Geometry: final body of the model. Coordinates: model frame, mm. Give positions to 0.01 mm unless a question says otherwise; leave off trailing zeros. Order: outer loops, then holes, each group sorted by start corner. A loop starts at its lowest first (then second) coordinate and runs counter-clockwise, first axis right, second up. Notation, with made-up numbers: (26.5, 1) -> (66.5, 1) arc R36 cw to (66.5, 40) -> close; hole circle Ø1 at (-0.5, -10). An arc over 180 degrees is marked (long way). One line per question, with ' | ' between items.
from build123d import *

# Parameters (mm, degrees)
SKETCH_1_R      = 1.65
EXTRUDE_1_DEPTH = 5
FILLET_1_R      = 2


with BuildPart() as part:
    # ｽｹｯﾁ1 → ﾎﾞｽ - 押し出し1 (new body)
    with BuildSketch(Plane.XY):
        Polygon((0, 0), (40, 0), (40, 15), (15, 60), (0, 60), align=None)
        with Locations((35, 7.5)):
            Circle(SKETCH_1_R, mode=Mode.SUBTRACT)
        with Locations((7.5, 7.5)):
            Circle(SKETCH_1_R, mode=Mode.SUBTRACT)
        with Locations((7.5, 22.5)):
            Circle(SKETCH_1_R, mode=Mode.SUBTRACT)
        with Locations((7.5, 52.5)):
            Circle(SKETCH_1_R, mode=Mode.SUBTRACT)
    extrude(amount=EXTRUDE_1_DEPTH)

    # ﾌｨﾚｯﾄ1
    fillet_1_edges = [part.edges().sort_by_distance(p)[0] for p in [
        (0, 60, 2.5),
        (15, 60, 2.5),
        (40, 15, 2.5),
        (40, 0, 2.5),
        (0, 0, 2.5),
    ]]
    fillet(fillet_1_edges, radius=FILLET_1_R)


solid = part.part
1) Section B-B on z = 2.55. Return loops of the section in (x, y), plus the area to 3 significant figures.
Check result:
outline: (0, 2) arc R2 ccw to (2, 0) -> (38, 0) arc R2 ccw to (40, 2) -> (40, 14.48) arc R2 ccw to (39.75, 15.45) -> (15.57, 58.97) arc R2 ccw to (13.82, 60) -> (2, 60) arc R2 ccw to (0, 58) -> close; hole circle Ø3.3 at (7.5, 7.5); hole circle Ø3.3 at (7.5, 22.5); hole circle Ø3.3 at (7.5, 52.5); hole circle Ø3.3 at (35, 7.5) | area: 1,800 mm^2
2) Section D-D on y = 22.5. Return loops of the section in (x, z), plus the area to 3 significant figures.
Check result:
outline: (0, 0) -> (5.85, 0) -> (5.85, 5) -> (0, 5) -> close; (9.15, 0) -> (35.83, 0) -> (35.83, 5) -> (9.15, 5) -> close | area: 163 mm^2
3) Section A-A on x = 7.5. Return loops of the section in (y, z).
Check result:
outline: (0, 0) -> (5.85, 0) -> (5.85, 5) -> (0, 5) -> close; (9.15, 0) -> (20.85, 0) -> (20.85, 5) -> (9.15, 5) -> close; (24.15, 0) -> (50.85, 0) -> (50.85, 5) -> (24.15, 5) -> close; (54.15, 0) -> (60, 0) -> (60, 5) -> (54.15, 5) -> close
4) Material intervals for probe 1 along Y at (x, z) = (7.5, 1.1); probe 2 along X at (y, z) = (9, 2.05); probe 3 along Y at (x, z) = (35, 2.75), sorted ascending. Write a range as from..to.
Check result:
probe 1: y = 0..5.85, 9.15..20.85, 24.15..50.85, 54.15..60 | probe 2: x = 0..6.81, 8.19..34.31, 35.69..40 | probe 3: y = 0..5.85, 9.15..24
5) Section C-C on x = 35. Return loops of the section in (y, z), plus the area to 4 significant figures.
Check result:
outline: (0, 0) -> (5.85, 0) -> (5.85, 5) -> (0, 5) -> close; (9.15, 0) -> (24, 0) -> (24, 5) -> (9.15, 5) -> close | area: 103.5 mm^2
6) Contact query for flat-ended pins moving along their axis: pin 1 Ø2 at (x, y) = (7.5, 22.5) entering from -Z; pin 2 Ø2 at (y, z) = (38, 4) entering from +X; pin 3 Ø2 at (x, z) = (34.5, 0.5) entering from +Y; pin 4 Ø3 at (y, z) = (52.5, 2) entering from +X. Output: stop coordinate, or through.
Check result:
pin 1: passes through | pin 2: stops at x = 27.78 | pin 3: stops at y = 26.7 | pin 4: stops at x = 20
